```python
from build123d import *

# Parameters (mm, degrees)
BOSS_EXTRUDE1_DEPTH = 12.7
FILLET1_R           = 6.35
HOLE1_D             = 3.175
HOLE1_DEPTH         = 12.7
HOLE1_CSINK_D       = 10.16
HOLE1_CSINK_ANGLE   = 82
HOLE1_TIP           = 0.953866233
HOLE2_D             = 3.175
HOLE2_DEPTH         = 31.75
HOLE2_CSINK_D       = 10.16
HOLE2_CSINK_ANGLE   = 82
HOLE2_TIP           = 0.953866233
CUT_EXTRUDE1_REACH  = 14.7
SKETCH6_W           = 88.9
SKETCH6_H           = 88.9
FILLET2_R           = 3.175
HOLE3_D             = 3.175
HOLE3_DEPTH         = 31.75
HOLE3_CSINK_D       = 10.16
HOLE3_CSINK_ANGLE   = 82
HOLE3_TIP           = 0.953866233


with BuildPart() as part:
    # Sketch1 → Boss-Extrude1 (new body)
    with BuildSketch(Plane.XY):
        Polygon((16.704465975, -230.262851166), (-93.295534025, -230.262851166), (-93.295534025, 250.666642396), (341.304465963, 250.666642396), (341.304465963, -230.262851166), (231.304465963, -230.262851166), (231.304465963, -60.262851166), (16.704465975, -60.262851166), align=None)
    extrude(amount=-BOSS_EXTRUDE1_DEPTH)

    # Fillet1
    fillet1_edges = [part.edges().sort_by_distance(p)[0] for p in [
        (286.304465963, -230.262851166, 0),
        (-38.295534025, -230.262851166, 0),
    ]]
    fillet(fillet1_edges, radius=FILLET1_R)

    # Hole1
    with Locations(Plane.XY):
        with Locations((218.604465963, -53.912851166), (331.779465963, -204.862851166), (331.779465963, 10.201895615), (331.779465963, 225.266642396), (331.779465963, 117.734269005), (331.779465963, -77.862851166), (164.983632635, 86.68320968), (290.800299298, 86.68320968), (237.654465963, -86.479517833), (237.654465963, -191.3461845), (124.004465969, 86.68320968), (124.004465969, 225.266642396), (124.004465969, -22.162851166), (10.354465975, -191.3461845), (10.354465975, -86.479517833), (-42.791367359, 86.68320968), (83.025299304, 86.68320968), (-83.770534025, -77.862851166), (-83.770534025, 117.734269005), (-83.770534025, 225.266642396), (-83.770534025, 10.201895615), (-83.770534025, -204.862851166), (124.004465969, -53.912851166), (29.404465975, -53.912851166)):
            CounterSinkHole(HOLE1_D / 2, HOLE1_CSINK_D / 2, depth=HOLE1_DEPTH, counter_sink_angle=HOLE1_CSINK_ANGLE)
            with Locations((0, 0, -(HOLE1_DEPTH + HOLE1_TIP / 2))):  # 118° drill point
                Cone(0, HOLE1_D / 2, HOLE1_TIP, mode=Mode.SUBTRACT)

    # Hole2
    with Locations(Plane(origin=(124.004465969, -215.287141225, 0), x_dir=(1, 0, 0), z_dir=(0, 0, 1))):
        with Locations((113.649999994, 128.807623392), (113.649999994, 23.940956725), (-94.599999994, 161.374290059), (94.599999994, 161.374290059), (0, 161.374290059), (0, 193.124290059), (0, 440.553783621), (0, 301.970350905), (40.979166666, 301.970350905), (166.795833328, 301.970350905), (207.774999994, 440.553783621), (207.774999994, 333.02141023), (207.774999994, 225.48903684), (207.774999994, 137.424290059), (207.774999994, 10.424290059), (-207.774999994, 10.424290059), (-207.774999994, 137.424290059), (-207.774999994, 225.48903684), (-207.774999994, 333.02141023), (-207.774999994, 440.553783621), (-166.795833328, 301.970350905), (-40.979166666, 301.970350905), (-113.649999994, 23.940956725), (-113.649999994, 128.807623392)):
            CounterSinkHole(HOLE2_D / 2, HOLE2_CSINK_D / 2, depth=HOLE2_DEPTH, counter_sink_angle=HOLE2_CSINK_ANGLE)
            with Locations((0, 0, -(HOLE2_DEPTH + HOLE2_TIP / 2))):  # 118° drill point
                Cone(0, HOLE2_D / 2, HOLE2_TIP, mode=Mode.SUBTRACT)

    # Sketch6 → Cut-Extrude1 (cut, up to next)
    with BuildSketch(Plane.XY, mode=Mode.PRIVATE) as cut_extrude1_sk1:
        with Locations((192.927465963, 27.76820968)):
            Rectangle(SKETCH6_W, SKETCH6_H)
    cut_extrude1_tool1 = extrude(cut_extrude1_sk1.sketch, amount=-CUT_EXTRUDE1_REACH, mode=Mode.PRIVATE) & part.part
    add(cut_extrude1_tool1.solids().sort_by_distance((192.927466, 27.76821, 0))[0], mode=Mode.SUBTRACT)

    # Fillet2
    fillet2_edges = [part.edges().sort_by_distance(p)[0] for p in [
        (148.477465963, -16.68179032, -6.35),
        (148.477465963, 72.21820968, -6.35),
        (237.377465963, 72.21820968, -6.35),
        (237.377465963, -16.68179032, -6.35),
    ]]
    fillet(fillet2_edges, radius=FILLET2_R)

    # Hole3
    with Locations(Plane(origin=(124.004465969, -215.287141225, 0), x_dir=(1, 0, 0), z_dir=(0, 0, 1))):
        with Locations((113.649999994, 128.807623392), (113.649999994, 23.940956725), (-94.599999994, 161.374290059), (94.599999994, 161.374290059), (0, 161.374290059), (0, 193.124290059), (0, 440.553783621), (0, 301.970350905), (40.979166666, 301.970350905), (166.795833328, 301.970350905), (207.774999994, 440.553783621), (207.774999994, 333.02141023), (207.774999994, 225.48903684), (207.774999994, 137.424290059), (207.774999994, 10.424290059), (-207.774999994, 10.424290059), (-207.774999994, 137.424290059), (-207.774999994, 225.48903684), (-207.774999994, 333.02141023), (-207.774999994, 440.553783621), (-166.795833328, 301.970350905), (-40.979166666, 301.970350905), (-113.649999994, 23.940956725), (-113.649999994, 128.807623392), (119.722999994, 198.605350905), (119.722999994, 271.630350905), (18.122999994, 198.605350905), (18.122999994, 271.630350905)):
            CounterSinkHole(HOLE3_D / 2, HOLE3_CSINK_D / 2, depth=HOLE3_DEPTH, counter_sink_angle=HOLE3_CSINK_ANGLE)
            with Locations((0, 0, -(HOLE3_DEPTH + HOLE3_TIP / 2))):  # 118° drill point
                Cone(0, HOLE3_D / 2, HOLE3_TIP, mode=Mode.SUBTRACT)


solid = part.part
```
Design review of the part built by this model. Coordinates are the model's own, in mm. A direction names the side the tool comes from. Round coordinates to 2 decimals unless told otherwise and drop trailing zeros. Write each loop counter-clockwise with the first axis right and the second up, starting at its lowest first coordinate (ties: lowest second). Pieces come first, ordered by that corner, then holes.
Item 1: We need section B-B on x = 69. Write out the cut boundary in (y, z), and give its area (3 significant figures).
Item 2: For probe 1 along Y at (x, z) = (10.5, -11.5); probe 2 along X at (y, z) = (-163, -9.25); probe 3 along Y at (x, z) = (9, -2), list the stretches that pass through material, from the lowest coordinate up.
Item 3: We need section C-C on z = -9.25. State how many separate pieces and enclosed holes the cut face has, and give its area (3 significant figures).
Item 4: Clearance check with flat-ended pins moving along their axes: pin 1 Ø4 at (x, y) = (331.78, 10.2) entering from +Z; pin 2 Ø1 at (x, z) = (39, -5.5) entering from -Y; pin 3 Ø5 at (x, y) = (243.73, 56.34) entering from +Z. State where each tip first meets the part, or that it passes through.
Item 5: We need section A-A on y = -110. Write out the cut boundary in (x, z).
Item 6: For faces 4 (the conical face through (-84.715, 119.216, -3.823)), 5 (the flat face through (148.477, 27, -6)), list the 3-axis set-ups (+Z, -Z, +X, -X, +Y, -Y) from which the entire face can be reached by the end or side of a thin tool; tool diameter is ignored.
Item 7: The part is to be moulded in two halves that separate along Y. For faces 1 (the flat face through (231.304, -146, -6)), 2 (the flat face through (126, -60.263, -6)), 3 (the conical face through (-84.72, -76.38, -3.82)), say which applies: +Y half, -Y half, draft (parallel to the pull), parting line (faces both ways), or undercut.
Returned:
1. outline: (-60.26, -12.7) - (250.67, -12.7) - (250.67, 0) - (-60.26, 0) - close
1. area: 3,950 mm2
2. probe 1: y = -230.26 to -192.93, -189.77 to -88.06, -84.9 to 250.67
2. probe 2: x = -93.3 to 16.7, 231.3 to 341.3
2. probe 3: y = -228.54 to -194.4, -188.29 to -89.53, -83.42 to 250.67
3. separate pieces: 1
3. enclosed holes: 29
3. area: 164,000 mm2
4. pin 1: stops at z = -3.54
4. pin 2: stops at y = -60.26
4. pin 3: stops at z = -2.96
5. outline: (-93.3, -12.7) - (16.7, -12.7) - (16.7, 0) - (-93.3, 0) - close; (231.3, -12.7) - (341.3, -12.7) - (341.3, 0) - (231.3, 0) - close
6. face 4: +Z
6. face 5: +Z, -Z
7. face 1: draft
7. face 2: -Y half
7. face 3: undercut
